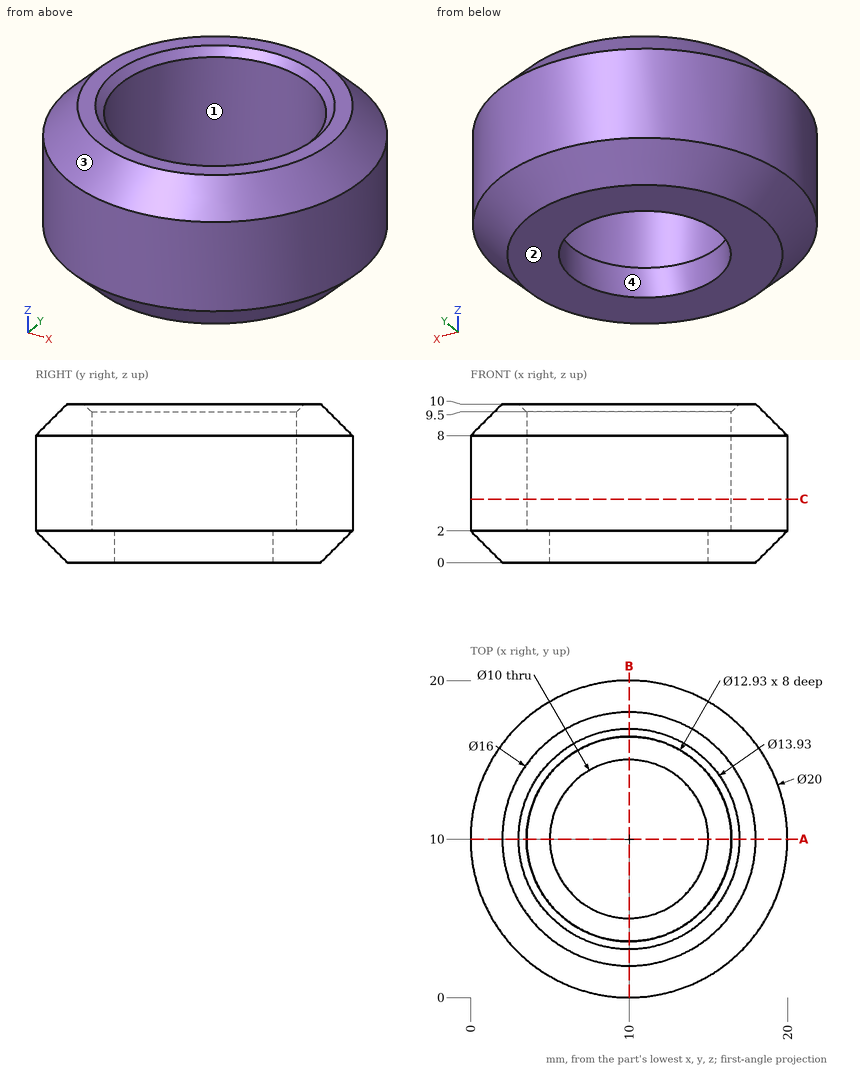
Input: dimensioned drawing with shaded views. Units: mm. Origin: part minimum x, y, z. Round coordinates to 2 decimals unless told otherwise and drop trailing zeros. Loops run counter-clockwise (first coordinate to the right, second up) from the corner with the lowest first, then second, coordinate; pieces in that order, holes last.
1) Material intervals for line 1 (Y direction, x = 10, z = 6) (3 decimals); line 2 (Y direction, x = 14.25, z = 3.75); line 3 (X direction, y = 11, z = 1.5), sorted ascending.
Ans:
line 1: y = 0 to 3.535, 16.465 to 20
line 2: y = 0.95 to 5.13, 14.87 to 19.05
line 3: x = 0.55 to 5.1, 14.9 to 19.45
2) Section query A-A on y = 10. Return the cut outline in (x, z) (3 decimals).
Ans:
outline: (0, 2) - (2, 0) - (5, 0) - (5, 2) - (3.535, 2) - (3.535, 9.5) - (3.035, 10) - (2, 10) - (0, 8) - close; (15, 0) - (18, 0) - (20, 2) - (20, 8) - (18, 10) - (16.965, 10) - (16.465, 9.5) - (16.465, 2) - (15, 2) - close
3) Section query C-C on z = 4. Return the cut outline in (x, y) (3 decimals).
Ans:
outline: circle Ø20 at (10, 10); hole circle Ø12.93 at (10, 10)
4) Pull-direction query (X, two-part tool) for the marked faces 1, 2, 3 and 4; classes: released by +X, released by -X, zero draft, split by the parting line, or undercut.
Ans:
face 1: undercut
face 2: zero draft
face 3: split by the parting line
face 4: undercut
5) Pin query (flat end, axial travel): pin 1 (3 mm diameter, centred on x = 17.5, y = 2.5, fed in from +Z); pin 2 (11.5 mm diameter, centred on x = 10, y = 10, fed in from -Z); pin 3 (3 mm diameter, centred on y = 3, z = 3, fed in from -X); pin 4 (2 mm diameter, centred on x = 11.5, z = 2.5, fed in from -Y). Return the tip coordinate at first contact, or that it passes through.
Ans:
pin 1: stops at z = 8.89
pin 2: stops at z = 0
pin 3: stops at x = 1.65
pin 4: stops at y = 0.01
